Verification items for this drawing (mm, ordinates from the low corner). Round coordinates to 2 decimals unless told otherwise and drop trailing zeros. Loops run counter-clockwise (first coordinate to the right, second up) from the corner with the lowest first, then second, coordinate; pieces in that order, holes last. Notation, with made-up numbers: M -37.75,-3.5 L -3.75,-3.5 A31 cw -3.75,21.5 Z; hole C 60,36.5 d9. An arc over 180 degrees is marked long. Answer as CSV lines item,"result".
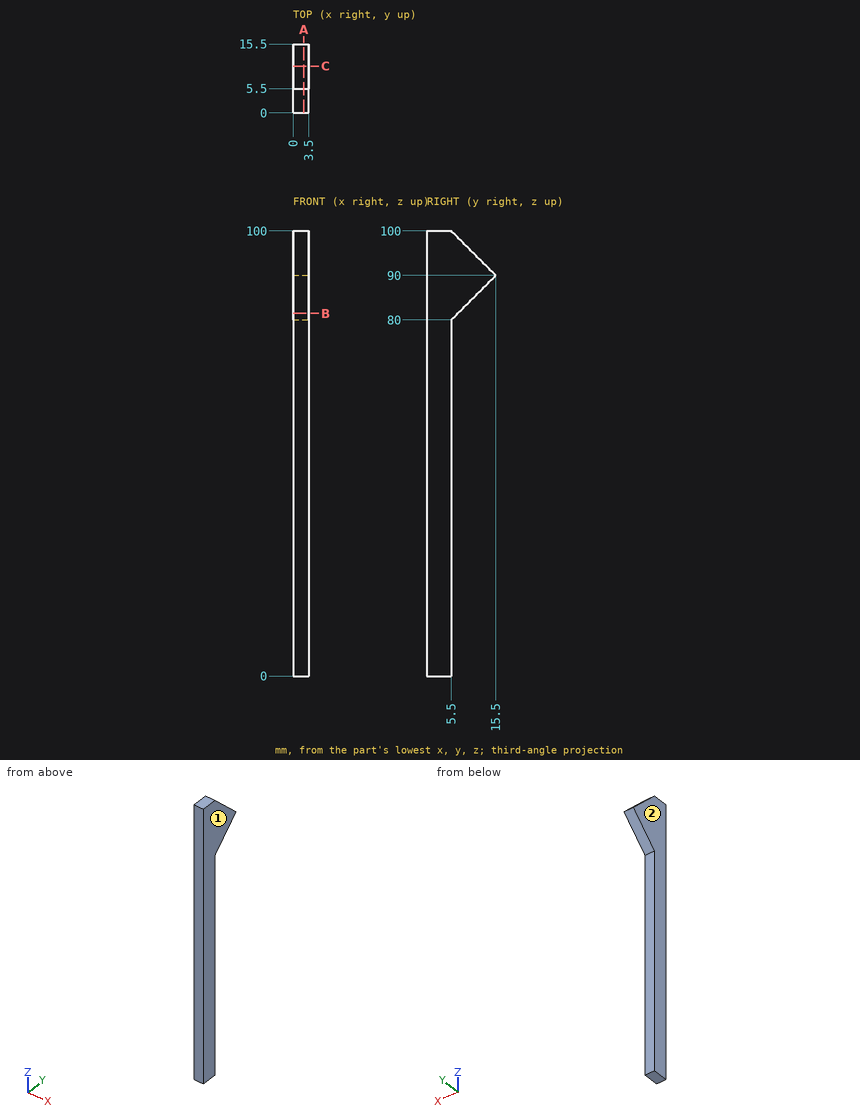
1) Draft check along X on the marked faces 1 and 2. Enter one of: +X half, -X half, draft (parallel to the pull), parting line (faces both ways), or undercut.
Here are the results:
face 1,"+X half"
face 2,"-X half"
2) Material ranges on probe 1 along Y at (x, z) = (0.45, 5.5); probe 2 along Z at (x, y) = (2, 12.25); probe 3 along Z at (x, y) = (1.25, 10), recorded low to high.
Here are the results:
probe 1,"y = 0 to 5.5"
probe 2,"z = 86.75 to 93.25"
probe 3,"z = 84.5 to 95.5"
3) Go/stop test with flat-tipped pins: pin 1 (1.5 mm diameter, centred on x = 1.5, y = 7.5, fed in from +Z); pin 2 (1.8 mm diameter, centred on x = 1, z = 52.5, fed in from +Y). Record where each tip stops, or that it passes through.
Here are the results:
pin 1,"stops at z = 98.75"
pin 2,"stops at y = 5.5"
4) Section check A-A (x = 2.4). Record the cut outline in (y, z), plus the area to 3 significant figures.
Here are the results:
outline,"M 0,0 L 5.5,0 L 5.5,80 L 15.5,90 L 5.5,100 L 0,100 Z"
area,"650 mm^2"
5) Section check C-C (y = 10.5). Record the cut outline in (x, z).
Here are the results:
outline,"M 0,85 L 3.5,85 L 3.5,95 L 0,95 Z"
6) Section check B-B (z = 81.5). Record the cut outline in (x, y), plus the area to 3 significant figures.
Here are the results:
outline,"M 0,0 L 3.5,0 L 3.5,7 L 0,7 Z"
area,"24.5 mm^2"
